Geometry check sheet. Reference: the model listing, model coordinates, mm. A direction names the side the tool comes from. Coordinates: 2 decimals unless noted, no trailing zeros. Write each loop counter-clockwise with the first axis right and the second up, starting at its lowest first coordinate (ties: lowest second). Pieces come first, ordered by that corner, then holes. Notation, with made-up numbers: (89.5, -37) -> (118.5, -37) arc R28 cw to (118.5, -12) -> close; hole circle Ø10 at (33, 80). An arc over 180 degrees is marked (long way). Answer in a Markdown table with one row per item. Add a question column.
1. Mould release check, pull along X, two halves, no side actions. Record for faces 1 (the flat face through (6, -20, 0)), 2 (the cylindrical face through (-14.985, 0.66, 3.451)), 3 (the cylindrical face through (-4.336, -19.524, 3.451)), 4 (the cylindrical face through (-29.97, 1.32, 4.93)): pulls with the +X half, pulls with the -X half, needs draft (parallel to the pull), parting line crosses it, or undercut.
2. Scan lines: L1, parallel to Y at x = 0, z = 1.5; L2, parallel to Y at x = 0, z = 7.75; L3, parallel to X at y = -1, z = 1.75. Record each from-to range of solid material in increasing order. Write a range as from..to.
3. Depth check by flat-ended pin: P1, Ø4, axis at y = -11.5, z = 7, coming from the -X side; P2, Ø4, axis at x = -8, z = 8, coming from the -Y side; P3, Ø6, axis at x = 20.5, z = 4, coming from the +Y side; P4, Ø18, axis at x = 0, y = 0, coming from the +Z side. Enter the tip coordinate at first touch or a pass-through.
4. Cross-section at D-D on x = -16. Record the cut outline in (y, z), and give its area (3 significant figures).
5. Cross-section at A-A on y = 0. Record the cut outline in (x, z), and give its area (3 significant figures).
6. Set-up check for faces 5 (the flat face through (13, 0, 10)), 6 (the flat face through (3, 15, 7)): record each of +Z, -Z, +X, -X, +Y, -Y from which the full face is reachable in a straight line by a thin tool's end or side.
7. Cross-section at C-C on z = 3. Record the cut outline in (x, y), and give its area (3 significant figures).
```python
from build123d import *

# Parameters (mm, degrees)
SKETCH_1_R          = 30
EXTRUDE_1_DEPTH     = 10
SKETCH_2_R          = 20
SKETCH_2_R_2        = 15
CUT_EXTRUDE_1_DEPTH = 7
SKETCH_3_R          = 10
CUT_EXTRUDE_2_DEPTH = 10


with BuildPart() as part:
    # 草图1 → 凸台-拉伸1 (new body)
    with BuildSketch(Plane.XY):
        Circle(SKETCH_1_R)
    extrude(amount=EXTRUDE_1_DEPTH)

    # 草图2 → 切除-拉伸1 (cut)
    with BuildSketch(Plane.XY):
        Circle(SKETCH_2_R)
        Circle(SKETCH_2_R_2, mode=Mode.SUBTRACT)
    extrude(amount=CUT_EXTRUDE_1_DEPTH, mode=Mode.SUBTRACT)

    # 草图3 → 切除-拉伸2 (cut)
    with BuildSketch(Plane(origin=(0, 0, 0), x_dir=(-1, 0, 0), z_dir=(0, 0, -1))):
        Circle(SKETCH_3_R)
    extrude(amount=-CUT_EXTRUDE_2_DEPTH, mode=Mode.SUBTRACT)


solid = part.part
```
Results found:
| question | item | result |
|---|---|---|
| 1 | face 1 | needs draft |
| 1 | face 2 | undercut |
| 1 | face 3 | undercut |
| 1 | face 4 | parting line crosses it |
| 2 | L1 | y = -30..-20, -15..-10, 10..15, 20..30 |
| 2 | L2 | y = -30..-10, 10..30 |
| 2 | L3 | x = -29.98..-19.97, -14.97..-9.95, 9.95..14.97, 19.97..29.98 |
| 3 | P1 | stops at x = -28.46 |
| 3 | P2 | stops at y = -29.39 |
| 3 | P3 | stops at y = 24.37 |
| 3 | P4 | passes through |
| 4 | outline | (-25.38, 0) -> (-12, 0) -> (-12, 7) -> (12, 7) -> (12, 0) -> (25.38, 0) -> (25.38, 10) -> (-25.38, 10) -> close |
| 4 | area | 340 mm^2 |
| 5 | outline | (-30, 0) -> (-20, 0) -> (-20, 7) -> (-15, 7) -> (-15, 0) -> (-10, 0) -> (-10, 10) -> (-30, 10) -> close; (10, 0) -> (15, 0) -> (15, 7) -> (20, 7) -> (20, 0) -> (30, 0) -> (30, 10) -> (10, 10) -> close |
| 5 | area | 330 mm^2 |
| 6 | face 5 | +Z, +X, -X, +Y, -Y |
| 6 | face 6 | -Z |
| 7 | outline | circle Ø60 at (0, 0); circle Ø30 at (0, 0); hole circle Ø40 at (0, 0); hole circle Ø20 at (0, 0) |
| 7 | area | 1,960 mm^2 |
